```python
from build123d import *

# Parameters (mm, degrees)
F0_R      = 3.2512
F1_DEPTH  = 4.4958
F2_R      = 5.2324
F3_DEPTH  = 6.35
F4_R      = 3.0226
F5_DEPTH  = 1.0922
F6_R      = 2.54
F7_DEPTH  = 23.7236
F9_W      = 15.0368
F9_H      = 0.508
F10_DEPTH = 7.7734
F11_R     = 0.254
F12_R     = 3.2512
F13_DEPTH = 0.762
F14_R     = 2.9464
F15_DEPTH = 0.762


with BuildPart() as f1:
    # F0 (on Right) → F1 (new body)
    with BuildSketch(Plane.YZ):
        Circle(F0_R)
    extrude(amount=F1_DEPTH)

    # F2 (on face) → F3 (join)
    with BuildSketch(Plane.YZ.offset(4.4958)):
        Circle(F2_R)
    extrude(amount=F3_DEPTH)

    # F4 (on face) → F5 (join)
    with BuildSketch(Plane.YZ.offset(10.8458)):
        Circle(F4_R)
    extrude(amount=F5_DEPTH)

    # F6 (on face) → F7 (join)
    with BuildSketch(Plane.YZ.offset(11.938)):
        Circle(F6_R)
    extrude(amount=F7_DEPTH)

    # F9 (on offset) → F10 (cut, through all)
    with BuildSketch(Plane.XY.offset(2.54)):
        with Locations((28.1432, 2.286)):
            Rectangle(F9_W, F9_H)
    extrude(amount=-F10_DEPTH, mode=Mode.SUBTRACT)

    # F11
    f11_edges = [f1.edges().sort_by_distance(p)[0] for p in [
        (35.6616, -2.54, 0),
    ]]
    fillet(f11_edges, radius=F11_R)

    # F12 (on face) → F13 (cut)
    with BuildSketch(Plane(origin=(0, 0, 0), x_dir=(0, -1, 0), z_dir=(-1, 0, 0))):
        Circle(F12_R)
    extrude(amount=-F13_DEPTH, mode=Mode.SUBTRACT)

    # F14 (on face) → F15 (join)
    with BuildSketch(Plane(origin=(0.762, 0, 0), x_dir=(0, -1, 0), z_dir=(-1, 0, 0))):
        Circle(F14_R)
    extrude(amount=F15_DEPTH)

    # F16 (on Front) → F17 (revolve)
    with BuildSketch(Plane.XZ):
        Polygon((0, 2.9464), (0.762, 2.9464), (0.762, 3.2512), align=None)
    revolve(axis=Axis((0.381, 0, 0), (1, 0, 0)))


solid = f1.part
```
Here's how the part is built. I have some questions about the finished solid (model axes, mm). A direction names the side the tool comes from. Round coordinates to 2 decimals unless told otherwise and drop trailing zeros. Loops run counter-clockwise (first coordinate to the right, second up) from the corner with the lowest first, then second, coordinate; pieces in that order, holes last. Notation, with made-up numbers: (-12.75, 49.25) -> (0.25, 49.25) arc R29 cw to (0.25, 82.25) -> close; hole circle Ø1 at (54, 33). An arc over 180 degrees is marked (long way). Answer as CSV lines item,"result". Start each with the question number.
1. Imagine slicing it at D-D on x = 16.5. Write out the boundary of the cut face in (y, z), plus the area to 3 significant figures.
2. I'm going to push flat-ended pins straight in: P1, Ø5, axis at x = 26.5, y = 1, coming from the +Z side; P2, Ø1.5, axis at x = 29.5, z = 0, coming from the +Y side; P3, Ø6, axis at x = 26.5, z = 4, coming from the -Y side. Where does each tip first touch, or does it pass through?
3. Imagine slicing it at B-B on y = 0. Write out the boundary of the cut face in (x, z).
4. Imagine slicing it at A-A on z = 0. Write out the boundary of the cut face in (x, y).
5. Imagine slicing it at C-C on x = 25. Write out the boundary of the cut face in (y, z).
6. I need wall thicknesses on probe 1 along X at (y, z) = (-4.25, 1); probe 2 along Z at (x, y) = (4, 0); probe 3 along Z at (x, y) = (16, 0). Which ranges of each line are inside material? Lowest first, please. Write a range as from..to.
7. For faces 1 (the face through (2.603, -0.423, 3.224)), 2 (the face through (28, 2.032, 0)), 3 (the face through (11.938, -2, 2)), which set-ups out of +Z, -Z, +X, -X, +Y, -Y let a thin tool reach every point of the face, with its end or its side?
Solution:
1,outline,"circle Ø5.08 at (0, 0)"
1,area,"20.3 mm²"
2,P1,"z = 2.54"
2,P2,"y = 2.03"
2,P3,"y = -2.33"
3,outline,"(0, -2.95) -> (0.76, -3.25) -> (4.5, -3.25) -> (4.5, -5.23) -> (10.85, -5.23) -> (10.85, -3.02) -> (11.94, -3.02) -> (11.94, -2.54) -> (35.41, -2.54) arc R0.25 ccw to (35.66, -2.29) -> (35.66, 2.29) arc R0.25 ccw to (35.41, 2.54) -> (11.94, 2.54) -> (11.94, 3.02) -> (10.85, 3.02) -> (10.85, 5.23) -> (4.5, 5.23) -> (4.5, 3.25) -> (0.76, 3.25) -> (0, 2.95) -> close"
4,outline,"(0, -2.95) -> (0.76, -3.25) -> (4.5, -3.25) -> (4.5, -5.23) -> (10.85, -5.23) -> (10.85, -3.02) -> (11.94, -3.02) -> (11.94, -2.54) -> (35.41, -2.54) arc R0.25 ccw to (35.66, -2.29) -> (35.66, 2.03) -> (20.62, 2.03) -> (20.62, 2.54) -> (11.94, 2.54) -> (11.94, 3.02) -> (10.85, 3.02) -> (10.85, 5.23) -> (4.5, 5.23) -> (4.5, 3.25) -> (0.76, 3.25) -> (0, 2.95) -> close"
5,outline,"(2.03, -1.52) -> (2.03, 1.52) arc R2.54 ccw (long way) to start"
6,probe 1,"4.5..10.85"
6,probe 2,"-3.25..3.25"
6,probe 3,"-2.54..2.54"
7,face 1,"-X"
7,face 2,"+Z, -Z, +X, +Y"
7,face 3,"+X"
